The model under review builds one solid part; all positions refer to its coordinate system, in mm. Face numbers are marked on the shaded views. A direction names the side the tool comes from. Round coordinates to 2 decimals unless told otherwise and drop trailing zeros. Loops run counter-clockwise (first coordinate to the right, second up) from the corner with the lowest first, then second, coordinate; pieces in that order, holes last. Notation, with made-up numbers: M 80.5,23.25 L 129.5,23.25 A15 ccw 129.5,48.25 Z; hole C 77,84.5 d3. An arc over 180 degrees is marked long. Use a Markdown table: item, result. Add a question column.
```python
from build123d import *

# Parameters (mm, degrees)
CONG_1_R = 1


with BuildPart() as part:
    # Esquisse1 → Révolution1 (revolve)
    with BuildSketch(Plane.XY, mode=Mode.PRIVATE) as r_volution1_sk:
        with BuildLine():
            Line((3, 1.2), (8, 1.2))
            Line((8, 1.2), (8, 4.7))
            Line((8, 4.7), (6.4, 4.7))
            Line((6.4, 4.7), (6.4, 10))
            Line((6.4, 10), (0, 10))
            Line((0, 10), (0, 0))
            ThreePointArc((0, 0), (1.615549442, 0.311126395), (3, 1.2))
        make_face()
    revolve(r_volution1_sk.sketch.rotate(Axis((0, 10, 0), (0, -1, 0)), 90), axis=Axis((0, 10, 0), (0, -1, 0)))

    # Congé1
    cong_1_edges = [part.edges().sort_by_distance(p)[0] for p in [
        (0, 10, -6.4),
        (0, 4.7, -8),
        (0, 1.2, -8),
    ]]
    fillet(cong_1_edges, radius=CONG_1_R)


solid = part.part
```
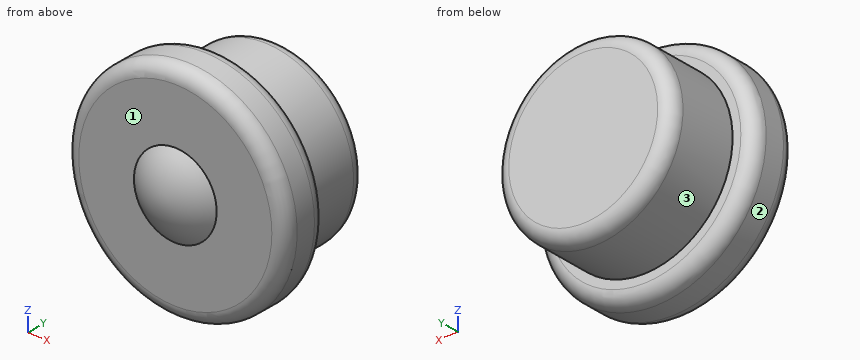
(1) For the marked faces 1, 2 and 3, list the 3-axis set-ups (+Z, -Z, +X, -X, +Y, -Y) from which the entire face can be reached by the end or side of a thin tool; tool diameter is ignored.
(2) Consider section B-B, the plane z = 0. Give the boundary of the cut face in (x, y).
(3) Consider section A-A, the plane x = 0. Give the boundary of the cut face in (y, z).
(4) To check wall thickness, follow probe 1 along Y at (x, z) = (-5.25, 0.5); probe 2 along Y at (x, z) = (5.5, -4.5); probe 3 along X at (y, z) = (6, -1.25). State the ranges of each line that lie inside material, in increasing order.
(5) Consider section D-D, the plane y = 1. Give the boundary of the cut face in (x, z).
(6) Consider section C-C, the plane y = 6. Give the boundary of the cut face in (x, z), then the cut area to 3 significant figures.
(7) Insertion check: pin 1 Ø3 at (x, y) = (3, 5.5) entering from +Z; pin 2 Ø1.5 at (y, z) = (1.5, -6) entering from +X; pin 3 Ø1.5 at (x, y) = (0.5, 4.5) entering from +Z; pin 4 Ø4 at (x, z) = (-0.5, -1) entering from -Y. Each pin has a flat end and moves straight along its axis. Give the tip position at first contact, or say it passes through.
Found:
| question | item | result |
|---|---|---|
| 1 | face 1 | -Y |
| 1 | face 2 | +Y, -Y |
| 1 | face 3 | +Y |
| 2 | outline | M -8,2.2 A1 ccw -7,1.2 L -3,1.2 A4.35 ccw 3,1.2 L 7,1.2 A1 ccw 8,2.2 L 8,3.7 A1 ccw 7,4.7 L 6.4,4.7 L 6.4,9 A1 ccw 5.4,10 L -5.4,10 A1 ccw -6.4,9 L -6.4,4.7 L -7,4.7 A1 ccw -8,3.7 Z |
| 3 | outline | M 1.2,-7 A1 ccw 2.2,-8 L 3.7,-8 A1 ccw 4.7,-7 L 4.7,-6.4 L 9,-6.4 A1 ccw 10,-5.4 L 10,5.4 A1 ccw 9,6.4 L 4.7,6.4 L 4.7,7 A1 ccw 3.7,8 L 2.2,8 A1 ccw 1.2,7 L 1.2,3 A4.35 ccw 1.2,-3 Z |
| 4 | probe 1 | y = 1.2 to 10 |
| 4 | probe 2 | y = 1.21 to 4.69 |
| 4 | probe 3 | x = -6.28 to 6.28 |
| 5 | outline | C 0,0 d5.55 |
| 6 | outline | C 0,0 d12.8 |
| 6 | area | 129 mm^2 |
| 7 | pin 1 | stops at z = 7.54 |
| 7 | pin 2 | stops at x = 5.87 |
| 7 | pin 3 | stops at z = 7.99 |
| 7 | pin 4 | stops at y = 0 |
